Geometry: final body of the model. Coordinates: model frame, mm. A direction names the side the tool comes from. Round coordinates to 2 decimals unless told otherwise and drop trailing zeros. Write each loop counter-clockwise with the first axis right and the second up, starting at its lowest first coordinate (ties: lowest second). Pieces come first, ordered by that corner, then holes. Notation, with made-up numbers: M -19.75,50.5 L 36.25,50.5 A24 ccw 36.25,60.5 Z; hole C -6.5,59.25 d8. An arc over 180 degrees is marked long. Answer as CSV lines item,"result". Start each with the question number.
Q1. First-contact query: pin 1 (1.6 mm diameter, centred on x = 0.5, z = 5.5, fed in from +Y); pin 2 (3 mm diameter, centred on y = 22, z = 4.5, fed in from +X); pin 3 (4 mm diameter, centred on x = 32, z = -8.5, fed in from -Y); pin 4 (1.5 mm diameter, centred on x = 28.5, y = 5.5, fed in from -Z). Flat tips, straight axial feed; report the tip coordinate or a pass-through.
Q2. Section query B-B on z = -5.75. Output: boundary loops of the cut face in (x, y).
Q3. Section query C-C on x = 22. Output: boundary loops of the cut face in (y, z), and give its area (3 significant figures).
Q4. Mould query, pull axis Y, two halves, no side actions, for faces 1 (the flat face through (37, 9, 0)), 2 (the cylindrical face through (13.83, 19.8, 0.86)), 3 (the flat face through (1, 9, 2.6)). Classes: pulls with the +Y half, pulls with the -Y half, needs draft (parallel to the pull), parting line crosses it, or undercut.
Q5. Reachability of faces 4 (the flat face through (1, 3.3, 6)), 5 (the flat face through (9, 29, -9)), 6 (the flat face through (31, 4.45, -5)) from +Z, -Z, +X, -X, +Y, -Y: full face, straight path, thin tool, end or side. Return the list, or none.
Q6. Section query D-D on y = 11. Output: boundary loops of the cut face in (x, z), and give its area (3 significant figures).
Q7. Section query A-A on y = 26.45. Output: boundary loops of the cut face in (x, z), and give its area (3 significant figures).
Q8. Ray query, probe 1 along Y at (x, z) = (8.25, -2.75); probe 2 along Y at (x, z) = (34, -6.25); probe 3 along Y at (x, z) = (7, 8). Return the intervals inside material, ascending.
```python
from build123d import *

# Parameters (mm, degrees)
CROQUIS1_W                 = 37
CROQUIS1_H                 = 18.9
SALIENTE_EXTRUIR1_DEPTH    = 9
VACIADO1_T                 = -2
CROQUIS2_W                 = 12.8
CROQUIS2_H                 = 12.3
CORTAR_EXTRUIR1_DEPTH      = 9
CROQUIS3_R                 = 2.5
SALIENTE_EXTRUIR2_DEPTH    = 12
CROQUIS4_R                 = 5
CORTAR_EXTRUIR2_DEPTH      = 9
REDONDEO1_R                = 3
CORTAR_EXTRUIR3_DEPTH      = 52.806394393
CORTAR_EXTRUIR3_DEPTH_BACK = 52.806394393
CROQUIS5_W                 = 8
CROQUIS5_H                 = 10
SALIENTE_EXTRUIR3_DEPTH    = 2
SALIENTE_EXTRUIR4_START    = 2
SALIENTE_EXTRUIR4_DEPTH    = 2
REDONDEO2_R                = 3


with BuildPart() as part:
    # Croquis1 → Saliente-Extruir1 (new body)
    with BuildSketch(Plane.XY):
        with Locations((18.5, 9.45)):
            Rectangle(CROQUIS1_W, CROQUIS1_H)
    extrude(amount=SALIENTE_EXTRUIR1_DEPTH)

    # Vaciado1
    vaciado1_openings = [part.faces().sort_by_distance(p)[0] for p in [
        (18.5, 9.45, 9),
    ]]
    offset(amount=VACIADO1_T, openings=vaciado1_openings, kind=Kind.INTERSECTION)

    # Croquis2 → Cortar-Extruir1 (cut)
    with BuildSketch(Plane.ZY):
        with Locations((9, 9.45)):
            Rectangle(CROQUIS2_W, CROQUIS2_H)
    extrude(amount=-CORTAR_EXTRUIR1_DEPTH, mode=Mode.SUBTRACT)

    # Croquis3 → Saliente-Extruir2 (add)
    with BuildSketch(Plane(origin=(0, 0, 0), x_dir=(-1, 0, 0), z_dir=(0, 0, -1))):
        Polygon((-16.5, -16.55), (0, -16.55), (0, 33.45), (-16.5, 33.45), (-16.5, 18.9), (-37, 18.9), (-37, 0), (-16.5, 0), align=None)
        with Locations((-8.25, 26.45)):
            Circle(CROQUIS3_R, mode=Mode.SUBTRACT)
        with Locations((-8.25, -7.55)):
            Circle(CROQUIS3_R, mode=Mode.SUBTRACT)
    extrude(amount=SALIENTE_EXTRUIR2_DEPTH)

    # Croquis4 → Cortar-Extruir2 (cut)
    with BuildSketch(Plane.XY):
        with Locations((8.25, -7.55)):
            Circle(CROQUIS4_R)
        with Locations((8.25, 26.45)):
            Circle(CROQUIS4_R)
    extrude(amount=-CORTAR_EXTRUIR2_DEPTH, mode=Mode.SUBTRACT)

    # Redondeo1
    redondeo1_edges = [part.edges().sort_by_distance(p)[0] for p in [
        (16.5, 33.45, -6),
        (16.5, 18.9, -6),
        (16.5, 0, -6),
        (16.5, -16.55, -6),
        (0, -16.55, -6),
        (0, 33.45, -6),
        (37, 18.9, -1.5),
        (37, 0, -1.5),
    ]]
    fillet(redondeo1_edges, radius=REDONDEO1_R)

    # Croquis5 → Cortar-Extruir3 (cut, two sides: drawn at the far end of the back side and taken through both)
    with BuildSketch(Plane.XY.offset(2).offset(-CORTAR_EXTRUIR3_DEPTH_BACK)):
        with Locations((31, 9.45)):
            Rectangle(CROQUIS5_W, CROQUIS5_H)
    extrude(amount=CORTAR_EXTRUIR3_DEPTH + CORTAR_EXTRUIR3_DEPTH_BACK, mode=Mode.SUBTRACT)

    # Croquis7 → Saliente-Extruir3 (add)
    with BuildSketch(Plane.XY.offset(9)):
        Polygon((0, 18.9), (12.3, 18.9), (12.3, 7.5), (20.514130343, 7.5), (20.514130343, 2), (20.514130343, 0), (12.3, 0), (0, 0), align=None)
    extrude(amount=SALIENTE_EXTRUIR3_DEPTH)

    # Croquis8 → Saliente-Extruir4 (add)
    with BuildSketch(Plane.XY.offset(9).offset(SALIENTE_EXTRUIR4_START)):
        with BuildLine():
            Line((35, 2), (20.514130343, 2))
            Line((20.514130343, 2), (20.514130343, 0))
            Line((20.514130343, 0), (34, 0))
            ThreePointArc((34, 0), (36.121320344, 0.878679656), (37, 3))
            Line((37, 3), (37, 15.9))
            ThreePointArc((37, 15.9), (36.121320344, 18.021320344), (34, 18.9))
            Line((34, 18.9), (12.3, 18.9))
            Line((12.3, 18.9), (12.3, 16.9))
            Line((12.3, 16.9), (20.389072173, 16.9))
            Line((20.389072173, 16.9), (35, 16.9))
            Line((35, 16.9), (35, 2))
        make_face()
        Polygon((20.389072173, 2), (20.514130343, 2), (35, 2), (35, 16.9), (20.389072173, 16.9), align=None)
    extrude(amount=-SALIENTE_EXTRUIR4_DEPTH)

    # Redondeo2
    redondeo2_edges = [part.edges().sort_by_distance(p)[0] for p in [
        (9.75, 18.9, 0),
        (9.75, 0, 0),
    ]]
    fillet(redondeo2_edges, radius=REDONDEO2_R)


solid = part.part
```
Entries:
1,pin 1,"stops at y = 18.9"
1,pin 2,"passes through"
1,pin 3,"stops at y = 0"
1,pin 4,"stops at z = 9"
2,outline,"M 0,-13.55 A3 ccw 3,-16.55 L 13.5,-16.55 A3 ccw 16.5,-13.55 L 16.5,-3 A3 cw 19.5,0 L 34,0 A3 ccw 37,3 L 37,15.9 A3 ccw 34,18.9 L 19.5,18.9 A3 cw 16.5,21.9 L 16.5,30.45 A3 ccw 13.5,33.45 L 3,33.45 A3 ccw 0,30.45 Z; hole C 8.25,-7.55 d10; hole C 8.25,26.45 d10; hole M 27,4.45 L 35,4.45 L 35,14.45 L 27,14.45 Z"
3,outline,"M 0,-12 L 18.9,-12 L 18.9,11 L 0,11 Z; hole M 2,2 L 16.9,2 L 16.9,9 L 2,9 Z"
3,area,"330 mm^2"
4,face 1,"needs draft"
4,face 2,"pulls with the +Y half"
4,face 3,"undercut"
5,face 4,"-X"
5,face 5,"+Z"
5,face 6,"-Z"
6,outline,"M 0,-12 L 27,-12 L 27,2 L 2,2 L 2,2.6 L 0,2.6 Z; M 0,9 L 12.3,9 L 12.3,11 L 0,11 Z; M 20.39,9 L 35,9 L 35,-12 L 37,-12 L 37,11 L 20.39,11 Z"
6,area,"479 mm^2"
7,outline,"M 0,-12 L 5.75,-12 L 5.75,-9 L 3.25,-9 L 3.25,0 L 0,0 Z; M 10.75,-12 L 16.5,-12 L 16.5,0 L 13.25,0 L 13.25,-9 L 10.75,-9 Z"
7,area,"93.0 mm^2"
8,probe 1,"y = -16.55 to -12.55, -2.55 to 21.45, 31.45 to 33.45"
8,probe 2,"y = 0 to 4.45, 14.45 to 18.9"
8,probe 3,"y = 0 to 2, 16.9 to 18.9"
